from build123d import *

# Parameters (mm, degrees)
SKETCH1_W           = 50
SKETCH1_H           = 50
SKETCH1_R           = 4.1
SKETCH1_R_2         = 3.1
BOSS_EXTRUDE1_DEPTH = 1.5
SKETCH2_R           = 5.6
SKETCH2_R_2         = 4.1
SKETCH2_R_3         = 4.6
SKETCH2_R_4         = 3.1
EXTRUDE_THIN1_DEPTH = 3
SKETCH3_W           = 70
SKETCH3_H           = 70
SKETCH3_R           = 2
SKETCH3_W_2         = 50
SKETCH3_H_2         = 50
BOSS_EXTRUDE2_DEPTH = 1


with BuildPart() as part:
    # Sketch1 → Boss-Extrude1 (new, symmetric)
    with BuildSketch(Plane(origin=(0, 0, 0), x_dir=(1, 0, 0), z_dir=(0, 1, 0))):
        with Locations((0, 25)):
            Rectangle(SKETCH1_W, SKETCH1_H)
        with Locations(Location((-12.426592672, 25, 0), (0, 0, 270))):
            Circle(SKETCH1_R, mode=Mode.SUBTRACT)
        with Locations(Location((-1.460779325, 25, 0), (0, 0, 270))):
            Circle(SKETCH1_R_2, mode=Mode.SUBTRACT)
        with Locations(Location((8.698724218, 25, 0), (0, 0, 270))):
            Circle(SKETCH1_R_2, mode=Mode.SUBTRACT)
    extrude(amount=BOSS_EXTRUDE1_DEPTH, both=True)

    # Sketch2 → Extrude-Thin1 (add)
    # profile 1 of 3: a face of its own
    with BuildSketch(Plane(origin=(0, 1.5, 0), x_dir=(1, 0, 0), z_dir=(0, 1, 0))):
        with Locations((-12.426592672, 25)):
            Circle(SKETCH2_R)
        with Locations((-12.426592672, 25)):
            Circle(SKETCH2_R_2, mode=Mode.SUBTRACT)
    # profile 2 of 3: a face of its own
    with BuildSketch(Plane(origin=(0, 1.5, 0), x_dir=(1, 0, 0), z_dir=(0, 1, 0))):
        with Locations((8.698724218, 25)):
            Circle(SKETCH2_R_3)
        with Locations((8.698724218, 25)):
            Circle(SKETCH2_R_4, mode=Mode.SUBTRACT)
    # profile 3 of 3: a face of its own
    with BuildSketch(Plane(origin=(0, 1.5, 0), x_dir=(1, 0, 0), z_dir=(0, 1, 0))):
        with Locations((-1.460779325, 25)):
            Circle(SKETCH2_R_3)
        with Locations((-1.460779325, 25)):
            Circle(SKETCH2_R_4, mode=Mode.SUBTRACT)
    extrude(amount=EXTRUDE_THIN1_DEPTH)

    # Sketch3 → Boss-Extrude2 (add)
    with BuildSketch(Plane.XZ.offset(1.5)):
        with Locations((0, -25)):
            Rectangle(SKETCH3_W, SKETCH3_H)
        with Locations(Location((-30, 5, 0), (0, 0, 270))):
            Circle(SKETCH3_R, mode=Mode.SUBTRACT)
        with Locations(Location((30, 5, 0), (0, 0, 270))):
            Circle(SKETCH3_R, mode=Mode.SUBTRACT)
        with Locations(Location((30, -55, 0), (0, 0, 270))):
            Circle(SKETCH3_R, mode=Mode.SUBTRACT)
        with Locations(Location((-30, -55, 0), (0, 0, 270))):
            Circle(SKETCH3_R, mode=Mode.SUBTRACT)
        with Locations((0, -25)):
            Rectangle(SKETCH3_W_2, SKETCH3_H_2, mode=Mode.SUBTRACT)
    extrude(amount=-BOSS_EXTRUDE2_DEPTH)


solid = part.part
Here's how the part is built. I have some questions about the finished solid (model axes, mm). A direction names the side the tool comes from. Give positions to 0.01 mm unless a question says otherwise; leave off trailing zeros. Order: outer loops, then holes, each group sorted by start corner. A loop starts at its lowest first (then second) coordinate and runs counter-clockwise, first axis right, second up. Notation, with made-up numbers: M -1,57 L 51,57 A16 ccw 51,85 Z; hole C 55,44.5 d3. An arc over 180 degrees is marked long. Answer as a JSON object with one key per item and string values. Group by question number.
1) Please list where these lines run through material, in increasing order: L1, parallel to X at y = 1.05, z = -25; L2, parallel to X at y = -1.1, z = 5; L3, parallel to X at y = 2.25, z = -24. Write a range as [from, to].
2) I'm going to push flat-ended pins straight in: pin 1 Ø1 at (y, z) = (1, -29.5) entering from +X; pin 2 Ø1.6 at (y, z) = (0.5, -34.5) entering from -X; pin 3 Ø5 at (x, z) = (-30, -55) entering from +Y. Where does each tip first touch, or does it pass through?
3) On a 3-axis mill with a long thin cutter (end or side, diameter ignored), from which of +Z, -Z, +X, -X, +Y, -Y can I reach the whole of each face in a straight line? I mean faces 5 (the cylindrical face through (11.17, 2.98, -28.88)), 6 (the flat face through (0, 1, -50)), 7 (the flat face through (-25, 1, -25)). Say none if no direction works.
4) We'd pull the mould along X, two halves only. Please class faces 1 (the flat face through (25, 1, -25)), 2 (the cylindrical face through (-32, -1, -55)), 3 (the cylindrical face through (-8.81, 1.46, -23.07)), 4 (the flat face through (-11.6, 4.5, -29.2)): pulls with the +X half, pulls with the -X half, needs draft (parallel to the pull), parting line crosses it, or undercut.
5) Suppose I cut it at C-C, the plane y = 0.7. Write out the boundary of the cut face in (x, z), plus the area to 3 significant figures.
6) Suppose I cut it at D-D, the plane x = -30. Write out the boundary of the cut face in (y, z), plus the area to 3 significant figures.
7) Suppose I cut it at A-A, the plane z = -55. Write out the boundary of the cut face in (x, y), plus the area to 3 significant figures.
8) Suppose I cut it at B-B, the plane x = 18.5. Write out the boundary of the cut face in (y, z), plus the area to 3 significant figures.
Results found:
{
 "1": {"L1": "[-25, -16.53], [-8.33, -4.56], [1.64, 5.6], [11.8, 25]", "L2": "[-35, -32], [-28, 28], [32, 35]", "L3": "[-17.94, -16.4], [-8.45, -6.92], [-5.95, -4.4], [1.47, 3.03], [4.21, 5.76], [11.63, 13.19]"},
 "2": {"pin 1": "x = 25", "pin 2": "x = -25", "pin 3": "y = -0.5"},
 "3": {"face 5": "+Y", "face 6": "-Z, +X, -X, +Y", "face 7": "+Z, -Z, -X, +Y"},
 "4": {"face 1": "pulls with the +X half", "face 2": "undercut", "face 3": "undercut", "face 4": "needs draft"},
 "5": {"outline": "M -25,-50 L 25,-50 L 25,0 L -25,0 Z; hole C -12.43,-25 d8.2; hole C -1.46,-25 d6.2; hole C 8.7,-25 d6.2", "area": "2,390 mm²"},
 "6": {"outline": "M -1.5,-60 L -0.5,-60 L -0.5,-57 L -1.5,-57 Z; M -1.5,-53 L -0.5,-53 L -0.5,3 L -1.5,3 Z; M -1.5,7 L -0.5,7 L -0.5,10 L -1.5,10 Z", "area": "62.0 mm²"},
 "7": {"outline": "M -35,-1.5 L -32,-1.5 L -32,-0.5 L -35,-0.5 Z; M -28,-1.5 L 28,-1.5 L 28,-0.5 L -28,-0.5 Z; M 32,-1.5 L 35,-1.5 L 35,-0.5 L 32,-0.5 Z", "area": "62.0 mm²"},
 "8": {"outline": "M -1.5,-60 L -0.5,-60 L -0.5,-50 L 1.5,-50 L 1.5,0 L -0.5,0 L -0.5,10 L -1.5,10 Z", "area": "170 mm²"}
}
